The model under review builds one solid part; all positions refer to its coordinate system, in mm. Face numbers are marked on the shaded views. Round coordinates to 2 decimals unless told otherwise and drop trailing zeros. Order: outer loops, then holes, each group sorted by start corner. A loop starts at its lowest first (then second) coordinate and runs counter-clockwise, first axis right, second up. Notation, with made-up numbers: (-25.5, 19) -> (17.5, 19) arc R14 ccw to (17.5, 24) -> close; hole circle Ø6 at (48, 18). An arc over 180 degrees is marked (long way). Return JSON: item names as keys, results as strings. Group by question number.
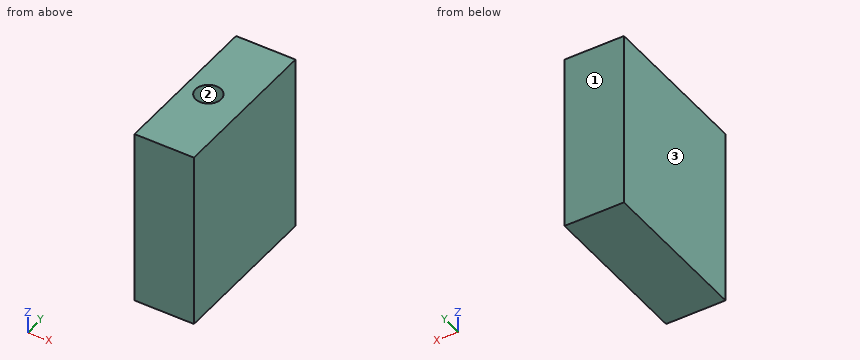
from build123d import *

# Parameters (mm, degrees)
CYLINDER002002001001001001001001008_R     = 0.97
CYLINDER002002001001001001001001008_DEPTH = 5
BOX006_W                                  = 4.5
BOX006_H                                  = 12
BOX006_DEPTH                              = 13.5


with BuildPart() as cylinder002002001001001001001001008:
    # Cylinder002002001001001001001001008 → Cylinder002002001001001001001001008 (new body)
    with BuildSketch(Plane(origin=(144.25, 12.8, 13.5), x_dir=(1, 0, 0), z_dir=(0, 0, 1))):
        Circle(CYLINDER002002001001001001001001008_R)
    extrude(amount=CYLINDER002002001001001001001001008_DEPTH)


with BuildPart() as cut013003021:
    # Box006 → Box006 (new body)
    with BuildSketch(Plane(origin=(142.5, 6.8, 5), x_dir=(1, 0, 0), z_dir=(0, 0, 1))):
        with Locations((2.25, 6)):
            Rectangle(BOX006_W, BOX006_H)
    extrude(amount=BOX006_DEPTH)

    # Cut013003021: cut Cylinder002002001001001001001001008
    add(cylinder002002001001001001001001008.part, mode=Mode.SUBTRACT)


solid = cut013003021.part
Item 1: Consider section C-C on z = 16.75. State the section outline as (x, y) points, plus the area to 3 significant figures.
Item 2: Insertion check: pin 1 Ø1.6 at (x, y) = (144.5, 13.5) entering from +Z. The pin has a flat end and moves straight along its axis. Give the tip position at first contact, or say it passes through.
Item 3: Consider section B-B on x = 144.25. State the section outline as (y, z) points, plus the area to 3 significant figures.
Item 4: Consider section A-A on y = 12.8. State the section outline as (x, z) points, plus the area to 4 significant figures.
Item 5: The part is to be moulded in two halves that separate along X. For the marked faces 1, 2 and 3, say which applies: +X half, -X half, draft (parallel to the pull), parting line (faces both ways), or undercut.
Item 6: Wall thickness on line 1 along Y through (x, z) = (144.25, 14.55); line 2 along Y through (x, z) = (143.85, 16.5): over which ranges is each line inside the solid? List them lowest first.
Values:
{
 "1": {"outline": "(142.5, 6.8) -> (147, 6.8) -> (147, 18.8) -> (142.5, 18.8) -> close; hole circle Ø1.94 at (144.25, 12.8)", "area": "51.0 mm^2"},
 "2": {"pin 1": "z = 18.5"},
 "3": {"outline": "(6.8, 5) -> (18.8, 5) -> (18.8, 18.5) -> (13.77, 18.5) -> (13.77, 13.5) -> (11.83, 13.5) -> (11.83, 18.5) -> (6.8, 18.5) -> close", "area": "152 mm^2"},
 "4": {"outline": "(142.5, 5) -> (147, 5) -> (147, 18.5) -> (145.22, 18.5) -> (145.22, 13.5) -> (143.28, 13.5) -> (143.28, 18.5) -> (142.5, 18.5) -> close", "area": "51.05 mm^2"},
 "5": {"face 1": "draft", "face 2": "undercut", "face 3": "-X half"},
 "6": {"line 1": "6.8 to 11.83, 13.77 to 18.8", "line 2": "6.8 to 11.92, 13.68 to 18.8"}
}
